Geometry check sheet. Reference: the model listing, model coordinates, mm. Give positions to 0.01 mm unless a question says otherwise; leave off trailing zeros. Loops run counter-clockwise (first coordinate to the right, second up) from the corner with the lowest first, then second, coordinate; pieces in that order, holes last. Notation, with made-up numbers: (-3.75, -19) - (18.25, -19) arc R8 ccw to (18.25, -14) - close; hole circle Ø11 at (84.5, -0.5). An arc over 180 degrees is marked (long way). Use a Markdown table: item, result. Add a question column.
1. Cross-section at D-D on x = -18. Enter the section's corners in (y, z).
2. Draft check along Z on faces 1 (the flat face through (-1, 12.7, -14)), 2 (the cylindrical face through (-2.75, 0.18, -12.4)), 3 (the flat face through (0, 0, -25.4)), 4 (the cylindrical face through (-35.27, -0.18, -20.19)). Enter one of: pulls with the +Z half, pulls with the -Z half, needs draft (parallel to the pull), parting line crosses it, or undercut.
3. Cross-section at A-A on x = 0. Enter the section's corners in (y, z), and give its area (3 significant figures).
4. Cross-section at B-B on y = 2.75. Enter the section's corners in (x, z).
5. Material ranges on L1, parallel to Z at x = 0, y = 10.75; L2, parallel to Z at x = 3.5, y = -9.5; L3, parallel to X at y = -3, z = 10, recorded low to high.
6. Cross-section at C-C on z = 0. Enter the section's corners in (x, y), and give its area (3 significant figures).
7. Depth check by flat-ended pin: P1, Ø6, axis at x = 17.5, y = 4, coming from the +Z side; P2, Ø8, axis at y = 7, z = 9, coming from the -X side; P3, Ø1, axis at y = -5, z = 19.5, coming from the +X side. Enter the tip coordinate at first touch or a pass-through.
from build123d import *

# Parameters (mm, degrees)
F0_R     = 12.7
F1_DEPTH = 12.7
F2_R     = 10.16


with BuildPart() as f1:
    # F0 (on Front) → F1 (new body, symmetric)
    with BuildSketch(Plane.XZ):
        Polygon((0, 50.8), (-43.994091, -25.4), (43.994091, -25.4), align=None)
        Circle(F0_R, mode=Mode.SUBTRACT)
    extrude(amount=F1_DEPTH, both=True)

    # F2
    f2_edges = [f1.edges().sort_by_distance(p)[0] for p in [
        (-43.994091, 0, -25.4),
        (43.994091, 0, -25.4),
        (0, 0, 50.8),
    ]]
    fillet(f2_edges, radius=F2_R)


solid = f1.part
Values found:
| question | item | result |
|---|---|---|
| 1 | outline | (-12.7, -25.4) - (12.7, -25.4) - (12.7, 19.62) - (-12.7, 19.62) - close |
| 2 | face 1 | needs draft |
| 2 | face 2 | undercut |
| 2 | face 3 | pulls with the -Z half |
| 2 | face 4 | parting line crosses it |
| 3 | outline | (-12.7, -25.4) - (12.7, -25.4) - (12.7, -12.7) - (-12.7, -12.7) - close; (-12.7, 12.7) - (12.7, 12.7) - (12.7, 40.64) - (-12.7, 40.64) - close |
| 3 | area | 1,030 mm2 |
| 4 | outline | (-35.2, -10.16) arc R10.16 ccw to (-26.4, -25.4) - (26.4, -25.4) arc R10.16 ccw to (35.2, -10.16) - (8.8, 35.56) arc R10.16 ccw to (-8.8, 35.56) - close; hole circle Ø25.4 at (0, 0) |
| 5 | L1 | z = -25.4 to -12.7, 12.7 to 40.64 |
| 5 | L2 | z = -25.4 to -12.21, 12.21 to 40.02 |
| 5 | L3 | x = -23.56 to -7.83, 7.83 to 23.56 |
| 6 | outline | (-29.33, -12.7) - (-12.7, -12.7) - (-12.7, 12.7) - (-29.33, 12.7) - close; (12.7, -12.7) - (29.33, -12.7) - (29.33, 12.7) - (12.7, 12.7) - close |
| 6 | area | 845 mm2 |
| 7 | P1 | stops at z = 25.69 |
| 7 | P2 | stops at x = -26.44 |
| 7 | P3 | stops at x = 18.36 |
